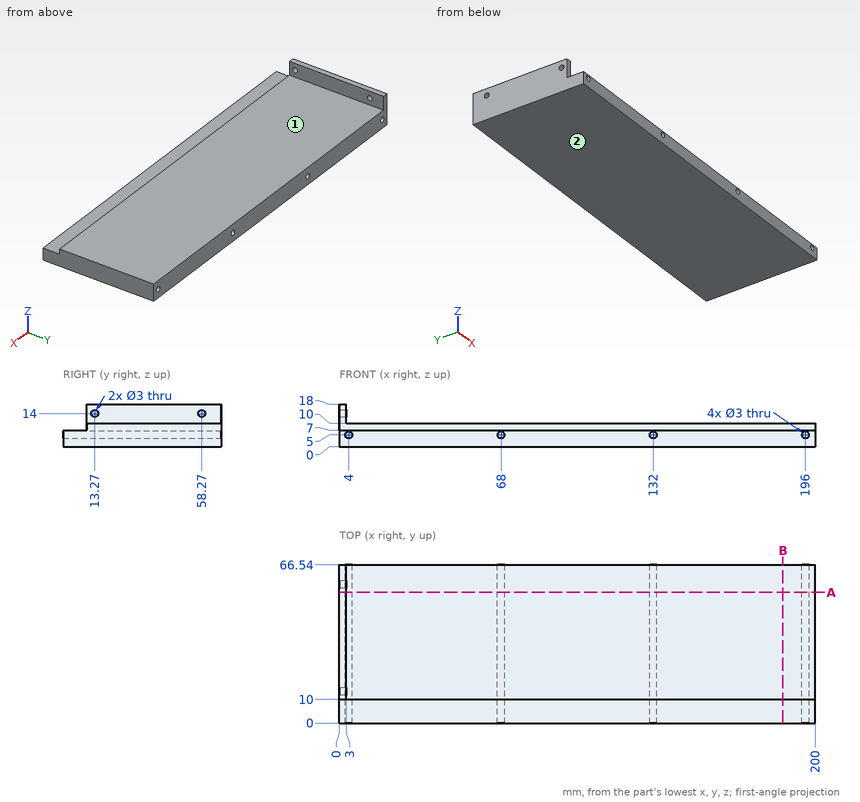
Can you work these out from the drawing? Everything is in mm from the part's minimum corner. A direction names the side the tool comes from. Give positions to 0.01 mm unless a question says otherwise; leave off trailing zeros. Loops run counter-clockwise (first coordinate to the right, second up) from the corner with the lowest first, then second, coordinate; pieces in that order, holes last. Notation, with made-up numbers: (65, 18) -> (72, 18) arc R5 cw to (72, 23) -> close; hole circle Ø2 at (65, 23.5). An arc over 180 degrees is marked (long way). Write item = value, one per line.
1) For the marked faces 1 and 2, which set-ups out of +Z, -Z, +X, -X, +Y, -Y let a thin tool reach every point of the face, with its end or its side?
Check result:
face_1 = +Z, +X, +Y, -Y
face_2 = -Z, +X, -X, +Y, -Y
2) Suppose I cut it at B-B on x = 186.5. Write out the boundary of the cut face in (y, z), then the cut area to 3 significant figures.
Check result:
outline = (0, 0) -> (66.54, 0) -> (66.54, 10) -> (10, 10) -> (10, 7) -> (0, 7) -> close
area = 635 mm2
3) Suppose I cut it at A-A on y = 55. Write out the boundary of the cut face in (x, z).
Check result:
outline = (0, 0) -> (200, 0) -> (200, 10) -> (3, 10) -> (3, 18) -> (0, 18) -> close; hole circle Ø3 at (4, 5); hole circle Ø3 at (68, 5); hole circle Ø3 at (132, 5); hole circle Ø3 at (196, 5)
4) I need wall thicknesses on L1, parallel to Y at x = 1.4, z = 14; L2, parallel to X at y = 14, z = 5; L3, parallel to Z at x = 4, y = 43. Which ranges of each line are inside material? Lowest first, please. Write a range as from..to.
Check result:
L1 = 10..11.77, 14.77..56.77, 59.77..66.54
L2 = 0..2.5, 5.5..66.5, 69.5..130.5, 133.5..194.5, 197.5..200
L3 = 0..3.5, 6.5..10
5) Will these pins go through, and if not, where does the flat tip stop? pin 1 (1.8 mm diameter, centred on y = 58.27, z = 14, fed in from +X); pin 2 (1 mm diameter, centred on y = 15.5, z = 14, fed in from -X); pin 3 (4 mm diameter, centred on y = 50, z = 15, fed in from +X); pin 4 (3 mm diameter, centred on x = 51, y = 50.5, fed in from +Z).
Check result:
pin_1 = through
pin_2 = 0
pin_3 = 3
pin_4 = 10
